```python
from build123d import *

# Parameters (mm, degrees)
SKETCH2_W            = 110
SKETCH2_H            = 30
BOSS_EXTRUDE2_DEPTH  = 10
SKETCH15_W           = 10
SKETCH15_H           = 15
BOSS_EXTRUDE9_DEPTH  = 60
SKETCH17_R           = 9.5
SKETCH17_R_2         = 7.5
EXTRUDE_THIN3_DEPTH  = 6
CUT_EXTRUDE4_START   = -5
CUT_EXTRUDE4_DEPTH   = 10
SKETCH19_W           = 10
SKETCH19_H           = 15
BOSS_EXTRUDE11_DEPTH = 100
SKETCH20_R           = 9.5
SKETCH20_R_2         = 7.5
EXTRUDE_THIN4_DEPTH  = 6
CUT_EXTRUDE5_START   = -5
CUT_EXTRUDE5_DEPTH   = 10
SKETCH21_W           = 10
SKETCH21_H           = 10
BOSS_EXTRUDE12_DEPTH = 70
SKETCH22_R           = 4
BOSS_EXTRUDE13_DEPTH = 100


# Read off the part's stored shape, not the designer's step: Cut-Extrude4, Cut-Extrude5
with BuildPart() as part:
    # Sketch2 → Boss-Extrude2 (new body)
    with BuildSketch(Plane(origin=(0, 0, 0), x_dir=(1, 0, 0), z_dir=(0, 1, 0))):
        with Locations((-5, 0)):
            Rectangle(SKETCH2_W, SKETCH2_H)
    extrude(amount=BOSS_EXTRUDE2_DEPTH)

    # Sketch15 → Boss-Extrude9 (add)
    with BuildSketch(Plane(origin=(0, 10, 0), x_dir=(1, 0, 0), z_dir=(0, 1, 0))):
        with Locations((-55, -7.5)):
            Rectangle(SKETCH15_W, SKETCH15_H)
    extrude(amount=BOSS_EXTRUDE9_DEPTH)

    # Sketch17 → Extrude-Thin3 (add, symmetric)
    with BuildSketch(Plane.ZY.offset(55)):
        with Locations((7.5, 70)):
            Circle(SKETCH17_R)
        with Locations((7.5, 70)):
            Circle(SKETCH17_R_2, mode=Mode.SUBTRACT)
    extrude(amount=EXTRUDE_THIN3_DEPTH, both=True)

    # Cut-Extrude4 outline → Cut-Extrude4 (cut)
    with BuildSketch(Plane.ZY.offset(55).offset(CUT_EXTRUDE4_START)):
        with BuildLine():
            ThreePointArc((0, 70), (7.5, 62.5), (15, 70))
            Line((15, 70), (0, 70))
        make_face()
    extrude(amount=CUT_EXTRUDE4_DEPTH, mode=Mode.SUBTRACT)

    # Sketch19 → Boss-Extrude11 (add)
    with BuildSketch(Plane(origin=(0, 10, 0), x_dir=(1, 0, 0), z_dir=(0, 1, 0))):
        with Locations((20, 7.5)):
            Rectangle(SKETCH19_W, SKETCH19_H)
    extrude(amount=BOSS_EXTRUDE11_DEPTH)

    # Sketch20 → Extrude-Thin4 (add, symmetric)
    with BuildSketch(Plane.ZY.offset(-20)):
        with Locations((-7.5, 110)):
            Circle(SKETCH20_R)
        with Locations((-7.5, 110)):
            Circle(SKETCH20_R_2, mode=Mode.SUBTRACT)
    extrude(amount=EXTRUDE_THIN4_DEPTH, both=True)

    # Cut-Extrude5 outline → Cut-Extrude5 (cut)
    with BuildSketch(Plane.ZY.offset(-20).offset(CUT_EXTRUDE5_START)):
        with BuildLine():
            ThreePointArc((-15, 110), (-7.5, 102.5), (0, 110))
            Line((0, 110), (-15, 110))
        make_face()
    extrude(amount=CUT_EXTRUDE5_DEPTH, mode=Mode.SUBTRACT)

    # Sketch21 → Boss-Extrude12 (add)
    with BuildSketch(Plane.XZ):
        with Locations((45, 0)):
            Rectangle(SKETCH21_W, SKETCH21_H)
    extrude(amount=BOSS_EXTRUDE12_DEPTH)

    # Sketch22 → Boss-Extrude13 (add)
    with BuildSketch(Plane.ZY.offset(-40)):
        with Locations(Location((0, -65, 0), (0, 0, 180))):
            Circle(SKETCH22_R)
    extrude(amount=BOSS_EXTRUDE13_DEPTH)


solid = part.part
```
Check sheet for the modelled part. Datum: model origin and axes. Units: mm. A direction names the side the tool comes from. Round coordinates to 2 decimals unless told otherwise and drop trailing zeros. Order: outer loops, then holes, each group sorted by start corner. A loop starts at its lowest first (then second) coordinate and runs counter-clockwise, first axis right, second up. Notation, with made-up numbers: (5, 74) - (57, 74) arc R29 ccw to (57, 96) - close; hole circle Ø2 at (-2, 15.5). An arc over 180 degrees is marked (long way). Answer as CSV lines item,"result". Start each with the question number.
1) Section check C-C (y = 110). Record the cut outline in (x, z).
2) Tool access check on faces 5 (the face through (-9.3, -61.095, 0.867)), 6 (the face through (45, -35, 5)), 7 (the face through (45, -35, -5)), 8 (the face through (-55, 37, 0)). Record the directions out of +Z, -Z, +X, -X, +Y, -Y that give a thin tool (end or side, any length) a straight path to the whole face; none if there is none.
3) Section check A-A (y = 70). Record the cut outline in (x, z), then the cut area to 3 significant figures.
4) Scan lines: probe 1 along Y at (x, z) = (-58.5, 7.5); probe 2 along Y at (x, z) = (16, -7); probe 3 along X at (y, z) = (9.5, -9). Record each from-to range of solid material in increasing order.
5) Draft check along X on faces 1 (the face through (-60, 32, 7)), 2 (the face through (25, 56, -7)), 3 (the face through (-6, 0, 0)), 4 (the face through (-49, 67, 0)). Enter one of: +X half, -X half, draft (parallel to the pull), parting line (faces both ways), or undercut.
6) Section check B-B (z = -7.5). Record the cut outline in (x, y).
7) Section check D-D (x = -42). Record the cut outline in (y, z).
8) Depth check by flat-ended pin: pin 1 (17 mm diameter, centred on y = 110, z = -7.5, fed in from +X); pin 2 (2 mm diameter, centred on y = 40, z = 2.5, fed in from +X); pin 3 (3 mm diameter, centred on y = -26, z = 0, fed in from -X); pin 4 (9.5 mm diameter, centred on y = 107.5, z = -7, fed in from +X). Enter the tip coordinate at first touch or a pass-through.
Determined:
1,outline,"(14, -17) - (26, -17) - (26, -15) - (14, -15) - close; (14, 0) - (26, 0) - (26, 2) - (14, 2) - close"
2,face 5,"-X"
2,face 6,"+Z, +X, -X, -Y"
2,face 7,"-Z, +X, -X, -Y"
2,face 8,"-Z, -X"
3,outline,"(-61, -2) - (-49, -2) - (-49, 0) - (-61, 0) - close; (-61, 15) - (-49, 15) - (-49, 17) - (-61, 17) - close; (15, -15) - (25, -15) - (25, 0) - (15, 0) - close"
3,area,"198 mm^2"
4,probe 1,"0 to 62.5, 77.5 to 79.5"
4,probe 2,"0 to 102.52, 117.48 to 119.49"
4,probe 3,"-60 to 50"
5,face 1,"-X half"
5,face 2,"+X half"
5,face 3,"draft"
5,face 4,"undercut"
6,outline,"(-60, 0) - (50, 0) - (50, 10) - (25, 10) - (25, 100.5) - (26, 100.5) - (26, 102.5) - (14, 102.5) - (14, 100.5) - (15, 100.5) - (15, 10) - (-60, 10) - close; (14, 117.5) - (26, 117.5) - (26, 119.5) - (14, 119.5) - close"
7,outline,"circle Ø8 at (-65, 0); (0, -15) - (10, -15) - (10, 15) - (0, 15) - close"
8,pin 1,"x = 26"
8,pin 2,"x = -50"
8,pin 3,"x = 40"
8,pin 4,"through"
